```python
from build123d import *

# Parameters (mm, degrees)
F0_W     = 24
F0_H     = 49
F1_DEPTH = 4
F2_R     = 7.5
F3_R     = 2.5
F4_DEPTH = 5


with BuildPart() as f1:
    # F0 (on Top) → F1 (new body)
    with BuildSketch(Plane.XY):
        Rectangle(F0_W, F0_H)
    extrude(amount=F1_DEPTH)

    # F2
    f2_edges = [f1.edges().sort_by_distance(p)[0] for p in [
        (12, -24.5, 2),
        (12, 24.5, 2),
    ]]
    fillet(f2_edges, radius=F2_R)

    # F3 (on face) → F4 (cut)
    with BuildSketch(Plane.XY.offset(4)):
        with Locations((4.5, 12.5)):
            Circle(F3_R)
        with Locations((4.5, -12.5)):
            Circle(F3_R)
    extrude(amount=-F4_DEPTH, mode=Mode.SUBTRACT)


solid = f1.part
```
Design review of the part built by this model. Coordinates are the model's own, in mm. Round coordinates to 2 decimals unless told otherwise and drop trailing zeros. Write each loop counter-clockwise with the first axis right and the second up, starting at its lowest first coordinate (ties: lowest second). Pieces come first, ordered by that corner, then holes. Notation, with made-up numbers: (69.25, 83) -> (73.25, 83) arc R4 ccw to (73.25, 89) -> close; hole circle Ø1 at (-37, -17). An arc over 180 degrees is marked (long way). Answer in a Markdown table with one row per item.
Q1. Clearance check with a flat-ended pin moving along its axis: pin 1 Ø8 at (x, y) = (4.5, -12.5) entering from +Z. State where the tip first meets the part, or that it passes through.
The answers:
| item | result |
|---|---|
| pin 1 | z = 4 |
Q2. To check wall thickness, follow L1, parallel to Y at x = 2.75, z = 1.85; L2, parallel to X at y = 17.5, z = 1.25; L3, parallel to Y at x = 9.5, z = 0.8. State the ranges of each line that lie inside material, in increasing order. Write a range as [from, to].
The answers:
| item | result |
|---|---|
| L1 | [-24.5, -14.29], [-10.71, 10.71], [14.29, 24.5] |
| L2 | [-12, 11.98] |
| L3 | [-22.59, 22.59] |
Q3. Take a section at A-A, the plane y = -12.5. State the section outline as (x, z) points.
The answers:
| item | result |
|---|---|
| outline | (-12, 0) -> (2, 0) -> (2, 4) -> (-12, 4) -> close; (7, 0) -> (12, 0) -> (12, 4) -> (7, 4) -> close |
Q4. Draft analysis for pull direction X (two halves, no side actions). For faces 1 (the face through (5.65, -14.72, 2.03)), 2 (the face through (9.745, -22.361, 2.028)), 3 (the face through (-12, 0, 2)), state which applies: +X half, -X half, draft (parallel to the pull), parting line (faces both ways), or undercut.
The answers:
| item | result |
|---|---|
| face 1 | undercut |
| face 2 | +X half |
| face 3 | -X half |
Q5. Take a section at D-D, the plane x = 8.5. State the section outline as (y, z) points.
The answers:
| item | result |
|---|---|
| outline | (-23.34, 0) -> (23.34, 0) -> (23.34, 4) -> (-23.34, 4) -> close |
Q6. Take a section at B-B, the plane z = 0.8. State the section outline as (x, y) points.
The answers:
| item | result |
|---|---|
| outline | (-12, -24.5) -> (4.5, -24.5) arc R7.5 ccw to (12, -17) -> (12, 17) arc R7.5 ccw to (4.5, 24.5) -> (-12, 24.5) -> close; hole circle Ø5 at (4.5, -12.5); hole circle Ø5 at (4.5, 12.5) |
Q7. Take a section at C-C, the plane x = 2.75. State the section outline as (y, z) points.
The answers:
| item | result |
|---|---|
| outline | (-24.5, 0) -> (-14.29, 0) -> (-14.29, 4) -> (-24.5, 4) -> close; (-10.71, 0) -> (10.71, 0) -> (10.71, 4) -> (-10.71, 4) -> close; (14.29, 0) -> (24.5, 0) -> (24.5, 4) -> (14.29, 4) -> close |
